from build123d import *

# Parameters (mm, degrees)
CBORE_FOR_M2_SHCS1_AT_2_COUNT = 2
CBORE_FOR_M2_SHCS1_AT_2_PITCH = 6.363961031
CBORE_FOR_M2_SHCS1_AT_3_COUNT = 2
CBORE_FOR_M2_SHCS1_AT_3_PITCH = 9
CBORE_FOR_M2_SHCS1_AT_4_COUNT = 2
CBORE_FOR_M2_SHCS1_AT_4_PITCH = 6.363961031


with BuildPart() as part:
    # Sketch1 → Revolve1 (revolve)
    with BuildSketch(Plane.XY):
        Polygon((0, 0), (0, 14.5), (2, 14.5), (2, 3.5), (8, 3.5), (8, 0), align=None)
    revolve(axis=Axis((0, 0, 0), (0, 1, 0)))

    # Sketch5 → CBORE for M2 SHCS1 (revolve, cut)
    with BuildSketch(Plane(origin=(0, 3.5, -4.5), x_dir=(0, 0, 1), z_dir=(1, 0, 0))):
        Polygon((0, 0), (0, 3.5), (1.1, 3.5), (1.1, 2), (2.2, 2), (2.2, 0.025), (2.225, 0), align=None)
    cbore_for_m2_shcs1 = revolve(axis=Axis((0, 9.85, -4.5), (0, -1, 0)), mode=Mode.SUBTRACT)

    # CBORE for M2 SHCS1 at 2: CBORE for M2 SHCS1 ×2
    with Locations(*[Vector(0.707106781, 0, 0.707106781) * (i * CBORE_FOR_M2_SHCS1_AT_2_PITCH) for i in range(1, CBORE_FOR_M2_SHCS1_AT_2_COUNT)]):
        add(cbore_for_m2_shcs1, mode=Mode.SUBTRACT)

    # CBORE for M2 SHCS1 at 3: CBORE for M2 SHCS1 ×2
    with Locations(*[(0, 0, i * CBORE_FOR_M2_SHCS1_AT_3_PITCH) for i in range(1, CBORE_FOR_M2_SHCS1_AT_3_COUNT)]):
        add(cbore_for_m2_shcs1, mode=Mode.SUBTRACT)

    # CBORE for M2 SHCS1 at 4: CBORE for M2 SHCS1 ×2
    with Locations(*[Vector(-0.707106781, 0, 0.707106781) * (i * CBORE_FOR_M2_SHCS1_AT_4_PITCH) for i in range(1, CBORE_FOR_M2_SHCS1_AT_4_COUNT)]):
        add(cbore_for_m2_shcs1, mode=Mode.SUBTRACT)


solid = part.part
Design review of the part built by this model. Coordinates are the model's own, in mm. A direction names the side the tool comes from. Round coordinates to 2 decimals unless told otherwise and drop trailing zeros. Write each loop counter-clockwise with the first axis right and the second up, starting at its lowest first coordinate (ties: lowest second). Pieces come first, ordered by that corner, then holes. Notation, with made-up numbers: M 29,29 L 79,29 A20 ccw 79,55 Z; hole C 61,52.5 d3. An arc over 180 degrees is marked long. One line per item, written item: value. Start each with the question number.
1. Take a section at A-A on x = 0. State the section outline as (y, z) points (3 decimals).
2. For faces 1 (the face through (3.41, 0.76, -0.14)), 2 (the face through (6.648, 2.501, -0.477)), list the 3-axis set-ups (+Z, -Z, +X, -X, +Y, -Y) from which the entire face can be reached by the end or side of a thin tool; tool diameter is ignored.
3. Clearance check with flat-ended pins moving along their axes: P1, Ø8, axis at y = 11, z = 5, coming from the +X side; P2, Ø4, axis at x = -4.5, z = 0, coming from the +Y side; P3, Ø8, axis at y = 11.5, z = 0, coming from the -X side. State where each tip first meets the part, or that it passes through.
4. Take a section at D-D on z = -4.5. State the section outline as (x, y) points (3 decimals).
5. To check wall thickness, follow probe 1 along Z at (x, y) = (0, 2.1); probe 2 along X at (y, z) = (0.75, 0). State the ranges of each line that lie inside material, in increasing order. Write a range as from..to.
6. Take a section at C-C on x = -4.5. State the section outline as (y, z) points (3 decimals), then the cut area to 3 significant figures.
7. Take a section at B-B on z = 0. State the section outline as (x, y) points (3 decimals).
8. Draft analysis for pull direction Z (two halves, no side actions). For faces 3 (the face through (-5.43, 0.76, 0.59)), 4 (the face through (-1.73, 1.73, 7.81)), 5 (the face through (3, 1.5, 0)), 6 (the face through (-2, 3.5, 2)), state which applies: pulls with the +Z half, pulls with the -Z half, needs draft (parallel to the pull), parting line crosses it, or undercut.
Computed:
1. outline: M 0,-8 L 3.5,-8 L 3.5,-6.725 L 3.475,-6.7 L 1.5,-6.7 L 1.5,-5.6 L 0,-5.6 Z; M 0,-3.4 L 1.5,-3.4 L 1.5,-2.3 L 3.475,-2.3 L 3.5,-2.275 L 3.5,-2 L 14.5,-2 L 14.5,2 L 3.5,2 L 3.5,2.275 L 3.475,2.3 L 1.5,2.3 L 1.5,3.4 L 0,3.4 Z; M 0,5.6 L 1.5,5.6 L 1.5,6.7 L 3.475,6.7 L 3.5,6.725 L 3.5,8 L 0,8 Z
2. face 1: +Y, -Y
2. face 2: +Y
3. P1: stops at x = 1.73
3. P2: stops at y = 1.5
3. P3: stops at x = -2
4. outline: M -6.614,0 L -1.1,0 L -1.1,1.5 L -2.2,1.5 L -2.2,3.475 L -2.225,3.5 L -6.614,3.5 Z; M 1.1,0 L 6.614,0 L 6.614,3.5 L 2.225,3.5 L 2.2,3.475 L 2.2,1.5 L 1.1,1.5 Z
5. probe 1: z = -8..-6.7, -2.3..2.3, 6.7..8
5. probe 2: x = -8..-5.6, -3.4..3.4, 5.6..8
6. outline: M 0,-6.614 L 3.5,-6.614 L 3.5,-2.225 L 3.475,-2.2 L 1.5,-2.2 L 1.5,-1.1 L 0,-1.1 Z; M 0,1.1 L 1.5,1.1 L 1.5,2.2 L 3.475,2.2 L 3.5,2.225 L 3.5,6.614 L 0,6.614 Z
6. area: 34.2 mm²
7. outline: M -8,0 L -5.6,0 L -5.6,1.5 L -6.7,1.5 L -6.7,3.475 L -6.725,3.5 L -8,3.5 Z; M -3.4,0 L 3.4,0 L 3.4,1.5 L 2.3,1.5 L 2.3,3.475 L 2.275,3.5 L 2,3.5 L 2,14.5 L -2,14.5 L -2,3.5 L -2.275,3.5 L -2.3,3.475 L -2.3,1.5 L -3.4,1.5 Z; M 5.6,0 L 8,0 L 8,3.5 L 6.725,3.5 L 6.7,3.475 L 6.7,1.5 L 5.6,1.5 Z
8. face 3: undercut
8. face 4: parting line crosses it
8. face 5: undercut
8. face 6: needs draft
